from build123d import *

# Parameters (mm, degrees)
BOSS_EXTRUDE1_DEPTH = 8
SKETCH2_W           = 15
SKETCH2_H           = 8
SKETCH2_W_2         = 8
SKETCH2_H_2         = 15
CUT_EXTRUDE1_DEPTH  = 160.750586853


with BuildPart() as part:
    # Sketch1 → Boss-Extrude1 (new body)
    with BuildSketch(Plane.XY):
        with BuildLine():
            Line((-82.5, -130), (82.5, -130))
            ThreePointArc((82.5, -130), (89.571067812, -127.071067812), (92.5, -120))
            Line((92.5, -120), (92.5, 120))
            ThreePointArc((92.5, 120), (89.571067812, 127.071067812), (82.5, 130))
            Line((82.5, 130), (-82.5, 130))
            ThreePointArc((-82.5, 130), (-89.571067812, 127.071067812), (-92.5, 120))
            Line((-92.5, 120), (-92.5, -120))
            ThreePointArc((-92.5, -120), (-89.571067812, -127.071067812), (-82.5, -130))
        make_face()
    extrude(amount=BOSS_EXTRUDE1_DEPTH)

    # Sketch2 → Cut-Extrude1 (cut, through all)
    with BuildSketch(Plane.XY.offset(8)):
        with Locations((0, 104)):
            Rectangle(SKETCH2_W, SKETCH2_H)
        with Locations((-40, 104)):
            Rectangle(SKETCH2_W, SKETCH2_H)
        with Locations((40, 104)):
            Rectangle(SKETCH2_W, SKETCH2_H)
        with Locations((-51.5, 47.5)):
            Rectangle(SKETCH2_W_2, SKETCH2_H_2)
        with Locations((-51.5, 77.5)):
            Rectangle(SKETCH2_W_2, SKETCH2_H_2)
        with Locations((51.5, 47.5)):
            Rectangle(SKETCH2_W_2, SKETCH2_H_2)
        with Locations((51.5, 77.5)):
            Rectangle(SKETCH2_W_2, SKETCH2_H_2)
    extrude(amount=-CUT_EXTRUDE1_DEPTH, mode=Mode.SUBTRACT)


solid = part.part
Could you check a few things on this model? Use its own coordinates, in mm. A direction names the side the tool comes from. Give positions to 0.01 mm unless a question says otherwise; leave off trailing zeros. Order: outer loops, then holes, each group sorted by start corner. A loop starts at its lowest first (then second) coordinate and runs counter-clockwise, first axis right, second up. Notation, with made-up numbers: (43.5, 57) - (84.5, 57) arc R28 cw to (84.5, 85) - close; hole circle Ø7 at (54.25, 5.5). An arc over 180 degrees is marked (long way). Return JSON: item names as keys, results as strings. Group by question number.
Q1. Thinking about a two-plate mould opening in X: for faces 3 (the face through (0, 108, 4)), 4 (the face through (-89.49, 127.15, 3.94)), 5 (the face through (-1, 2, 0)), 6 (the face through (51, 40, 4)), which applies, pulls with the +X half, pulls with the -X half, needs draft (parallel to the pull), parting line crosses it, or undercut?
Q2. Suppose I cut it at A-A, the plane x = 43.5. Please give me the cut outline in (y, z), and give its area (3 significant figures).
Q3. Which directions (+Z, -Z, +X, -X, +Y, -Y) give clear straight access to the entire face, cutting with the end or side of a thin tool? Please do faces 1 (the face through (-1, -130, 4)), 2 (the face through (-47.5, 104, 4)).
Q4. Please list where these lines run through material, in increasing order: line 1 along X through (y, z) = (46.5, 7.5); line 2 along Y through (x, z) = (-49, 4.25); line 3 along Y through (x, z) = (5, 3.5). Write a range as [from, to].
Q5. Suppose I cut it at B-B, the plane z = 3. State how many separate pieces and enclosed holes the cut face has, and give its area (3 significant figures).
Resolved:
{
 "1": {"face 3": "undercut", "face 4": "pulls with the -X half", "face 5": "needs draft", "face 6": "undercut"},
 "2": {"outline": "(-130, 0) - (100, 0) - (100, 8) - (-130, 8) - close; (108, 0) - (130, 0) - (130, 8) - (108, 8) - close", "area": "2,020 mm2"},
 "3": {"face 1": "+Z, -Z, +X, -X, -Y", "face 2": "+Z, -Z"},
 "4": {"line 1": "x = [-92.5, -55.5], [-47.5, 47.5], [55.5, 92.5]", "line 2": "y = [-130, 40], [55, 70], [85, 130]", "line 3": "y = [-130, 100], [108, 130]"},
 "5": {"separate pieces": "1", "enclosed holes": "7", "area": "47,200 mm2"}
}
